The listing builds one solid part. Answer for the finished solid, in the listing's coordinates (mm). Face numbers are marked on the shaded views. A direction names the side the tool comes from. Coordinates: 2 decimals unless noted, no trailing zeros. Write each loop counter-clockwise with the first axis right and the second up, starting at its lowest first coordinate (ties: lowest second). Pieces come first, ordered by that corner, then holes. Notation, with made-up numbers: M 85.25,-29.5 L 144.25,-29.5 A17 cw 144.25,-7.5 Z; hole C -13,76 d4. An arc over 180 degrees is marked long. Write item = value, one per line. Start each with the question number.
```python
from build123d import *


with BuildPart() as f1:
    # F0 (on Front) → F1 (revolve)
    with BuildSketch(Plane.XZ):
        Polygon((10.6, 4.802996), (6.6, 4.802996), (6.6, 2.802996), (8.6, 2.802996), align=None)
        Polygon((8.6, 2.802996), (6.6, 2.802996), (6.6, -2.197004), (6.6, -3.697004), (6.6, -5.197004), (10.6, -5.197004), (8.6, -3.197004), align=None)
        Polygon((6.6, -3.697004), (6.6, -2.197004), (4.6, -2.197004), (4.6, -5.197004), (6.6, -5.197004), align=None)
    revolve(axis=Axis((0, 0, 0.589413), (0, 0, 1)))


solid = f1.part
```
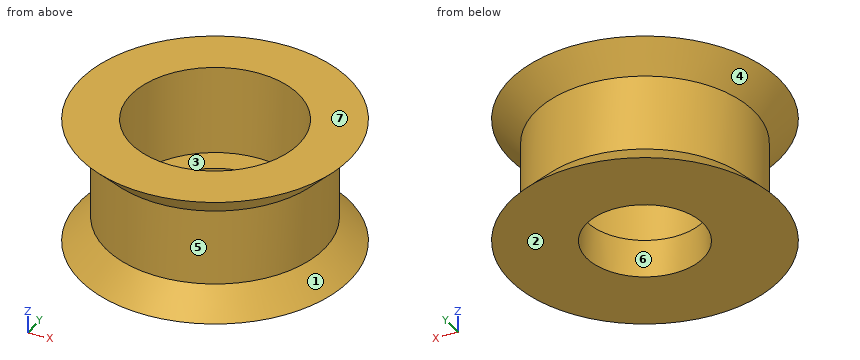
1. The part is cut by section A-A, the plane x = 0. Write down the section's boundary in (y, z).
2. Straight lines are drawn through the part: L1, parallel to Y at x = 0, z = -2.9; L2, parallel to Y at x = 0, z = 0.5; L3, parallel to X at y = 2.75, z = 1.5. For each, find the intervals that lie inside material, in ascending order. Write a range as [from, to].
3. Each of these flat-tipped pins is pushed along its axis until it touches: pin 1 (2 mm diameter, centred on y = 4, z = -4, fed in from -X); pin 2 (1 mm diameter, centred on x = -4.5, z = 2, fed in from +Y); pin 3 (4 mm diameter, centred on x = 5, z = 1.5, fed in from +Y); pin 4 (10.5 mm diameter, centred on x = -2.5, y = 1.5, fed in from +Z). Where does it stop, or does it pass through?
4. For a pull along Z with two mould halves and no side action, classify the marked faces 4, 5, 6 and 7 as pulls with the +Z half, pulls with the -Z half, needs draft (parallel to the pull), parting line crosses it, or undercut.
5. For the marked faces 1, 2 and 3, determine the directions among +Z, -Z, +X, -X, +Y, -Y from which every point of the face is accessible in a straight line to the end or side of a thin tool.
6. The part is cut by section D-D, the plane z = -4. Write down the section's boundary in (x, y), and give its area (3 significant figures).
7. The part is cut by section C-C, the plane z = 1.5. Write down the section's boundary in (x, y).
Solution:
q1.outline = M -10.6,-5.2 L -4.6,-5.2 L -4.6,-2.2 L -6.6,-2.2 L -6.6,4.8 L -10.6,4.8 L -8.6,2.8 L -8.6,-3.2 Z; M 4.6,-5.2 L 10.6,-5.2 L 8.6,-3.2 L 8.6,2.8 L 10.6,4.8 L 6.6,4.8 L 6.6,-2.2 L 4.6,-2.2 Z
q2.L1 = [-8.6, -4.6], [4.6, 8.6]
q2.L2 = [-8.6, -6.6], [6.6, 8.6]
q2.L3 = [-8.15, -6], [6, 8.15]
q3.pin_1 = -9.67
q3.pin_2 = 7.61
q3.pin_3 = 8.11
q3.pin_4 = 4.8
q4.face_4 = undercut
q4.face_5 = undercut
q4.face_6 = needs draft
q4.face_7 = pulls with the +Z half
q5.face_1 = none
q5.face_2 = -Z, +X, -X, +Y, -Y
q5.face_3 = +Z
q6.outline = C 0,0 d18.81; hole C 0,0 d9.2
q6.area = 211 mm^2
q7.outline = C 0,0 d17.2; hole C 0,0 d13.2
